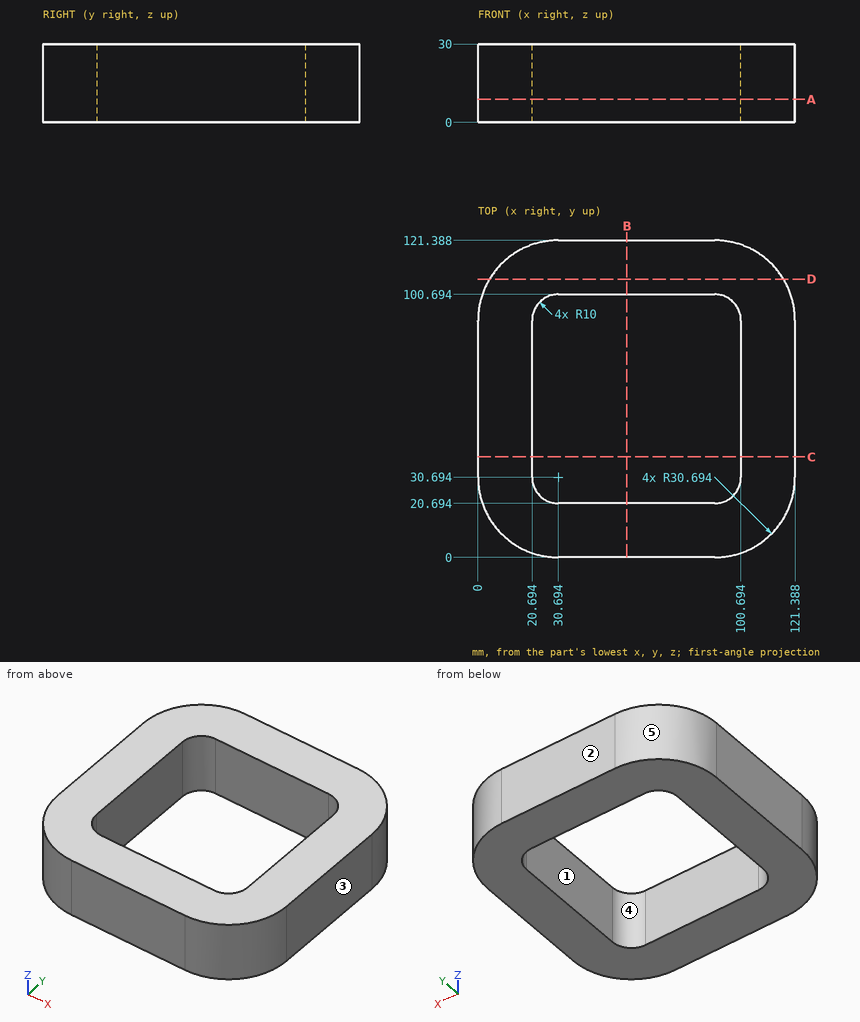
Study the drawing (mm; zero at the part's minimum x, y, z) and answer. A direction names the side the tool comes from. Coordinates: 2 decimals unless noted, no trailing zeros. Write each loop counter-clockwise with the first axis right and the second up, starting at its lowest first coordinate (ties: lowest second). Pieces come first, ordered by that corner, then holes.
Q1. The mould has two halves that part along X. Classify the marked faces 1, 2 and 3: released by +X, released by -X, zero draft, split by the parting line, or undercut.
Returned:
face 1: undercut
face 2: zero draft
face 3: released by +X
Q2. Which of the six approach directions +Z, -Z, +X, -X, +Y, -Y give full straight-line access (tool end or side, diameter ignored) to the marked faces 4 and 5?
Returned:
face 4: +Z, -Z
face 5: +Z, -Z, -X, +Y
Q3. Given P1, Ø5, axis at x = 91.5, z = 24, coming from the +Y side; P2, Ø5, axis at y = 93.5, z = 20.5, coming from the -X side, each flat-ended and moving along its own axis, determine where each tip first touches the part or whether it passes through.
Returned:
P1: stops at y = 121.39
P2: stops at x = 0
Q4. Section D-D, the plane y = 106.5 is taken. Write down the section's boundary in (x, z) (1 decimal), then the cut area to 3 significant figures.
Returned:
outline: (4.4, 0) - (117, 0) - (117, 30) - (4.4, 30) - close
area: 3,380 mm2
Q5. Section B-B, the plane x = 57 is taken. Write down the section's boundary in (y, z), then the cut area to 3 significant figures.
Returned:
outline: (0, 0) - (20.69, 0) - (20.69, 30) - (0, 30) - close; (100.69, 0) - (121.39, 0) - (121.39, 30) - (100.69, 30) - close
area: 1,240 mm2
Q6. Section A-A, the plane z = 8.75 is taken. Write down the section's boundary in (x, y), then the cut area to 3 significant figures.
Returned:
outline: (0, 30.69) arc R30.69 ccw to (30.69, 0) - (90.69, 0) arc R30.69 ccw to (121.39, 30.69) - (121.39, 90.69) arc R30.69 ccw to (90.69, 121.39) - (30.69, 121.39) arc R30.69 ccw to (0, 90.69) - close; hole (20.69, 30.69) arc R10 ccw to (30.69, 20.69) - (90.69, 20.69) arc R10 ccw to (100.69, 30.69) - (100.69, 90.69) arc R10 ccw to (90.69, 100.69) - (30.69, 100.69) arc R10 ccw to (20.69, 90.69) - close
area: 7,610 mm2
Q7. Find the intervals of material crossed by line 1 along X through (y, z) = (75, 8.75); line 2 along X through (y, z) = (24.5, 14.75) (1 decimal), in increasing order.
Returned:
line 1: x = 0 to 20.69, 100.69 to 121.39
line 2: x = 0.6 to 22.8, 98.5 to 120.8
